Check sheet for the modelled part. Datum: model origin and axes. Units: mm. A direction names the side the tool comes from. Give positions to 0.01 mm unless a question says otherwise; leave off trailing zeros. Loops run counter-clockwise (first coordinate to the right, second up) from the corner with the lowest first, then second, coordinate; pieces in that order, holes last. Notation, with made-up numbers: (35, -26.5) - (59, -26.5) arc R19 ccw to (59, -12.5) - close; hole circle Ø3 at (30.5, 86.25). An arc over 180 degrees is marked (long way). Use one line per item in the form item = value.
from build123d import *

# Parameters (mm, degrees)
BOSS_EXTRU_2_DEPTH      = 5
ENL_V_MAT_EXTRU_1_DEPTH = 5
ESQUISSE4_R             = 10.133372482
ENL_V_MAT_EXTRU_2_DEPTH = 10


with BuildPart() as part:
    # Esquisse1 → Boss.-Extru.2 (new body)
    with BuildSketch(Plane.XY):
        Polygon((-81.043275043, -69.971346705), (68.956724957, -69.971346705), (68.956724957, -60.737835253), (73.956724957, -60.737835253), (73.956724957, 39.262164747), (68.956724957, 39.262164747), (68.956724957, 45.028653295), (58.956724957, 45.028653295), (58.956724957, 50.028653295), (-71.043275043, 50.028653295), (-71.043275043, 45.028653295), (-81.043275043, 45.028653295), (-81.043275043, 40.028653295), (-86.043275043, 40.028653295), (-86.043275043, -59.971346705), (-81.043275043, -59.971346705), align=None)
    extrude(amount=BOSS_EXTRU_2_DEPTH)

    # Esquisse3 → Enlèv. mat.-Extru.1 (cut)
    with BuildSketch(Plane.XY.offset(5)):
        Polygon((-16.543275043, 37.028653295), (-16.543275043, -5.971346705), (4.456724957, -5.971346705), (4.456724957, 37.028653295), (-1.043275043, 37.028653295), (-1.043275043, 42.028653295), (-6.043275043, 42.028653295), (-11.043275043, 42.028653295), (-11.043275043, 37.028653295), align=None)
    extrude(amount=-ENL_V_MAT_EXTRU_1_DEPTH, mode=Mode.SUBTRACT)

    # Esquisse4 → Enlèv. mat.-Extru.2 (cut)
    with BuildSketch(Plane.XY.offset(5)):
        with Locations((-35.098604503, -26.562111751)):
            Circle(ESQUISSE4_R)
    extrude(amount=-ENL_V_MAT_EXTRU_2_DEPTH, mode=Mode.SUBTRACT)


solid = part.part
Item 1: Gauge pin test, flat ends, axial feed: P1, Ø2.5, axis at x = -84.5, z = 3, coming from the -Y side; P2, Ø2.5, axis at x = -82.5, z = 3.5, coming from the +Y side; P3, Ø2.5, axis at y = 47.5, z = 3.5, coming from the +X side. Record the tip position at first contact, or that the pin passes through.
Answer block:
P1 = -59.97
P2 = 40.03
P3 = 58.96
Item 2: Thickness scan on L1, parallel to X at y = 16.5, z = 4.2; L2, parallel to Y at x = -12, z = 4.55; L3, parallel to Y at x = -11, z = 2.1. Record the ranges inside material, lowest first.
Answer block:
L1 = -86.04 to -16.54, 4.46 to 73.96
L2 = -69.97 to -5.97, 37.03 to 50.03
L3 = -69.97 to -5.97, 42.03 to 50.03
Item 3: Mould release check, pull along Y, two halves, no side actions. Record for faces 1 (the face through (-7, -69.971, 2)), 2 (the face through (-42.567, -19.713, 2.535)), 3 (the face through (58.957, 47, 2)), 4 (the face through (-5, 50.029, 2)): released by +Y, released by -Y, zero draft, split by the parting line, or undercut.
Answer block:
face_1 = released by -Y
face_2 = undercut
face_3 = zero draft
face_4 = released by +Y
Item 4: Section check B-B on x = -33.5. Record the boundary of the cut face in (y, z).
Answer block:
outline = (-69.97, 0) - (-36.57, 0) - (-36.57, 5) - (-69.97, 5) - close; (-16.56, 0) - (50.03, 0) - (50.03, 5) - (-16.56, 5) - close
Item 5: Access from +Z, -Z, +X, -X, +Y, -Y to the whole of each face (thin tool, end or side, straight path). Record for faces 5 (the face through (68.957, -65, 2)), 6 (the face through (-81.043, 43, 2)), 7 (the face through (-14, 37.029, 3)), 8 (the face through (68.957, 42, 2)), 9 (the face through (-84, -59.971, 2)).
Answer block:
face_5 = +Z, -Z, +X, -Y
face_6 = +Z, -Z, -X, +Y
face_7 = +Z, -Z
face_8 = +Z, -Z, +X, +Y
face_9 = +Z, -Z, -X, -Y
Item 6: Section check C-C on z = 3.9. Record the boundary of the cut face in (x, y).
Answer block:
outline = (-86.04, -59.97) - (-81.04, -59.97) - (-81.04, -69.97) - (68.96, -69.97) - (68.96, -60.74) - (73.96, -60.74) - (73.96, 39.26) - (68.96, 39.26) - (68.96, 45.03) - (58.96, 45.03) - (58.96, 50.03) - (-71.04, 50.03) - (-71.04, 45.03) - (-81.04, 45.03) - (-81.04, 40.03) - (-86.04, 40.03) - close; hole circle Ø20.27 at (-35.1, -26.56); hole (-16.54, -5.97) - (4.46, -5.97) - (4.46, 37.03) - (-1.04, 37.03) - (-1.04, 42.03) - (-11.04, 42.03) - (-11.04, 37.03) - (-16.54, 37.03) - close
Item 7: Section check A-A on y = 22. Record the boundary of the cut face in (x, z).
Answer block:
outline = (-86.04, 0) - (-16.54, 0) - (-16.54, 5) - (-86.04, 5) - close; (4.46, 0) - (73.96, 0) - (73.96, 5) - (4.46, 5) - close
